The drawing under review shows one solid part. Ordinate dimensions are in mm from its lowest x, y, z. Coordinates: 2 decimals unless noted, no trailing zeros. Loops run counter-clockwise (first coordinate to the right, second up) from the corner with the lowest first, then second, coordinate; pieces in that order, holes last.
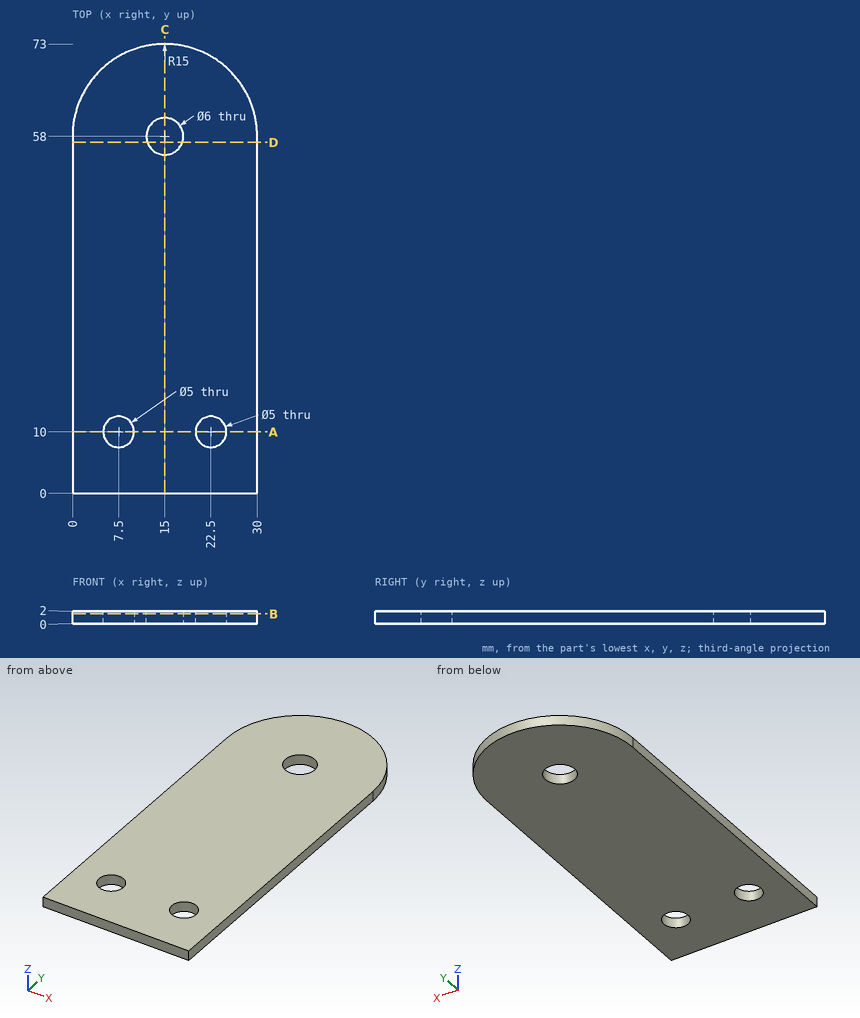
Q1. Take a section at A-A, the plane y = 10. Write out the cut boundary in (x, z).
Q2. For line 1 (Y direction, x = 21, z = 1.05); line 2 (Y direction, x = 12.5, z = 0.7); line 3 (X direction, y = 60, z = 0.75), list the stretches that pass through material, from the lowest coordinate up.
Q3. Take a section at B-B, the plane z = 1.6. Write out the cut boundary in (x, y).
Q4. Take a section at C-C, the plane x = 15. Write out the cut boundary in (y, z), then the cut area to 3 significant figures.
Q5. Take a section at D-D, the plane y = 57. Write out the cut boundary in (x, z).
Entries:
1. outline: (0, 0) - (5, 0) - (5, 2) - (0, 2) - close; (10, 0) - (20, 0) - (20, 2) - (10, 2) - close; (25, 0) - (30, 0) - (30, 2) - (25, 2) - close
2. line 1: y = 0 to 8, 12 to 71.75
2. line 2: y = 0 to 56.34, 59.66 to 72.79
2. line 3: x = 0.13 to 12.76, 17.24 to 29.87
3. outline: (0, 0) - (30, 0) - (30, 58) arc R15 ccw to (0, 58) - close; hole circle Ø5 at (7.5, 10); hole circle Ø6 at (15, 58); hole circle Ø5 at (22.5, 10)
4. outline: (0, 0) - (55, 0) - (55, 2) - (0, 2) - close; (61, 0) - (73, 0) - (73, 2) - (61, 2) - close
4. area: 134 mm2
5. outline: (0, 0) - (12.17, 0) - (12.17, 2) - (0, 2) - close; (17.83, 0) - (30, 0) - (30, 2) - (17.83, 2) - close
